Part model, mm, in its own coordinate system. Face numbers are marked on the shaded views. A direction names the side the tool comes from. Round coordinates to 2 decimals unless told otherwise and drop trailing zeros. Loops run counter-clockwise (first coordinate to the right, second up) from the corner with the lowest first, then second, coordinate; pieces in that order, holes last. Notation, with made-up numbers: (40.5, 45) -> (57.5, 45) arc R27 ccw to (57.5, 82) -> close; hole circle Ø6 at (6, 17.5). An arc over 180 degrees is marked (long way). Use a Markdown table: item, result. Add a question column.
Item 1: Flat gauge pins, fed straight in: pin 1 (4 mm diameter, centred on x = 14.5, z = -1.5, fed in from -Y); pin 2 (4 mm diameter, centred on y = 34.5, z = -1, fed in from -X); pin 3 (13.5 mm diameter, centred on x = 0, y = -50, fed in from +Z); pin 4 (1.5 mm diameter, centred on x = -4, z = -1.5, fed in from -Y). Where does each tip first touch, or does it go through?
Item 2: Cut at D-D, the plane y = 54. List the corners of the cut face in (x, z).
Item 3: Cut at A-A, the plane y = 0. List the corners of the cut face in (x, z), plus the area to 3 significant figures.
Item 4: Which spindle directions (+Z, -Z, +X, -X, +Y, -Y) get a long thin tool onto all of the face, cutting with end or side? Do the marked faces 5 and 6. Say none if no direction does.
Item 5: Cut at B-B, the plane x = 41. List the corners of the cut face in (y, z).
Item 6: Two-plate mould, pull along X, no slides. Class the marked faces 1, 2, 3 and 4: pulls with the +X half, pulls with the -X half, needs draft (parallel to the pull), parting line crosses it, or undercut.
Item 7: Cut at C-C, the plane z = 1. State how many separate pieces and enclosed holes the cut face has, plus the area to 3 significant figures.
Item 8: Probe line 1 (Y direction, x = 0, z = 0.75); line 2 (Y direction, x = 0, z = -1.5); line 3 (Y direction, x = 50, z = 1.25). List the from-to ranges inside material, lowest first. Write a range as [from, to].
```python
from build123d import *

# Parameters (mm, degrees)
F0_R        = 11.1
F1_DEPTH    = 3.5
F2_T        = 2.5
F2_T3_DEPTH = 12


# Not quite as in the source:
# - a shell that OpenCascade refuses in one call is made with other operations: the cavity is built on its own and cut out


with BuildPart() as f1:
    # F0 (on Top) → F1 (new body, symmetric)
    with BuildSketch(Plane.XY):
        with BuildLine():
            Line((29.2040910572, 29.1611850262), (15, 50))
            ThreePointArc((15, 50), (0, 35), (-15, 50))
            Line((-15, 50), (-29.2040910572, 29.1611850262))
            Line((-29.2040910572, 29.1611850262), (-50, 15))
            ThreePointArc((-50, 15), (-39.3933982822, 10.6066017178), (-35, 0))
            ThreePointArc((-35, 0), (-39.3933982822, -10.6066017178), (-50, -15))
            Line((-50, -15), (-29.2040910572, -29.1611850262))
            Line((-29.2040910572, -29.1611850262), (-15, -50))
            ThreePointArc((-15, -50), (0, -35), (15, -50))
            Line((15, -50), (29.2040910572, -29.1611850262))
            Line((29.2040910572, -29.1611850262), (50, -15))
            ThreePointArc((50, -15), (35, 0), (50, 15))
            Line((50, 15), (29.2040910572, 29.1611850262))
        make_face()
        Circle(F0_R, mode=Mode.SUBTRACT)
        with BuildLine():
            ThreePointArc((-15, 50), (0, 35), (15, 50))
            ThreePointArc((15, 50), (0, 65), (-15, 50))
        make_face()
        with Locations((0, 50)):
            Circle(F0_R, mode=Mode.SUBTRACT)
        with BuildLine():
            ThreePointArc((65, 0), (60.6066017178, 10.6066017178), (50, 15))
            ThreePointArc((50, 15), (35, 0), (50, -15))
            ThreePointArc((50, -15), (60.6066017178, -10.6066017178), (65, 0))
        make_face()
        with Locations((50, 0)):
            Circle(F0_R, mode=Mode.SUBTRACT)
        with BuildLine():
            ThreePointArc((-15, -50), (0, -65), (15, -50))
            ThreePointArc((15, -50), (0, -35), (-15, -50))
        make_face()
        with Locations((0, -50)):
            Circle(F0_R, mode=Mode.SUBTRACT)
        with BuildLine():
            ThreePointArc((-35, 0), (-39.3933982822, 10.6066017178), (-50, 15))
            ThreePointArc((-50, 15), (-65, 0), (-50, -15))
            ThreePointArc((-50, -15), (-39.3933982822, -10.6066017178), (-35, 0))
        make_face()
        with Locations((-50, 0)):
            Circle(F0_R, mode=Mode.SUBTRACT)
    extrude(amount=F1_DEPTH, both=True)

    # F2: shell of thickness 2.5, made by hand


with BuildPart() as f2_core1:
    # F2_t2: copy of F1
    add(f1.part)

    # the walls: a layer under each face that stays
    f2_faces = [f2_core1.faces().sort_by_distance(p)[0] for p in [
        (39.6020455286, -22.0805925131, 0),
        (22.1020455286, -39.5805925131, 0),
        (0, -65, 0),
        (-22.1020455286, -39.5805925131, 0),
        (-39.6020455286, -22.0805925131, 0),
        (-65, 0, 0),
        (-39.6020455286, 22.0805925131, 0),
        (-22.1020455286, 39.5805925131, 0),
        (0, 65, 0),
        (22.1020455286, 39.5805925131, 0),
        (39.6020455286, 22.0805925131, 0),
        (-61.1, 0, 0),
        (-11.1, -50, 0),
        (38.9, 0, 0),
        (-11.1, 50, 0),
        (-11.1, 0, 0),
        (65, 0, 0),
        (-37.1428571429, -18.5714285714, -3.5),
    ]]
    thicken(f2_faces, amount=-F2_T, mode=Mode.SUBTRACT)

    # F2_s4 → F2_t3 (cut)
    with BuildSketch(Plane.XY.offset(-6)):
        Polygon((50.0140713144, -15.0456639326), (48.5928685595, -12.933606739), (49.2296264469, -12.5), (50, -12.5), align=None)
        Polygon((29.2388199891, -29.1959295426), (27.7969596167, -27.0947917651), (27.4052462259, -27.3615329699), (27.1383293075, -27.753126649), align=None)
        Polygon((15.0456576175, -50.0140805838), (12.9342382503, -48.5919416228), (12.5, -49.2290123454), (12.5, -50), align=None)
        Polygon((-15.0456576175, -50.0140805838), (-12.5, -50), (-12.5, -49.2290123454), (-12.9342382503, -48.5919416228), align=None)
        Polygon((-29.2388199891, -29.1959295426), (-27.1383293075, -27.753126649), (-27.4052462259, -27.3615329699), (-27.7969596167, -27.0947917651), align=None)
        Polygon((-50.0140713144, -15.0456639326), (-48.5928685595, -12.933606739), (-49.2296264469, -12.5), (-50, -12.5), align=None)
        Polygon((-50.0140713144, 15.0456639326), (-50, 12.5), (-49.2296264469, 12.5), (-48.5928685595, 12.933606739), align=None)
        Polygon((-29.2388199891, 29.1959295426), (-27.7969596167, 27.0947917651), (-27.4052462259, 27.3615329699), (-27.1383293075, 27.753126649), align=None)
        Polygon((-15.0456576175, 50.0140805838), (-12.9342382503, 48.5919416228), (-12.5, 49.2290123454), (-12.5, 50), align=None)
        Polygon((15.0456576175, 50.0140805838), (12.5, 50), (12.5, 49.2290123454), (12.9342382503, 48.5919416228), align=None)
        Polygon((29.2388199891, 29.1959295426), (27.1383293075, 27.753126649), (27.4052462259, 27.3615329699), (27.7969596167, 27.0947917651), align=None)
        Polygon((50.0140713144, 15.0456639326), (48.5928685595, 12.933606739), (49.2296264469, 12.5), (50, 12.5), align=None)
    extrude(amount=F2_T3_DEPTH, mode=Mode.SUBTRACT)


with BuildPart() as f1_1:
    add(f1.part)

    # what is left inside the walls is the cavity
    f2_cavity = [f2_core1.part.solids().sort_by_distance(p)[0] for p in [
        (0, -15.95435, 3.475),
    ]]
    add(f2_cavity, mode=Mode.SUBTRACT)


solid = f1_1.part
```
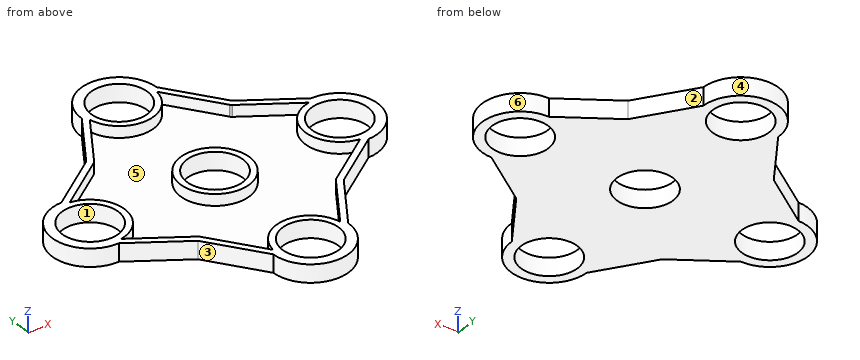
A:
| question | item | result |
|---|---|---|
| 1 | pin 1 | stops at y = -58.29 |
| 1 | pin 2 | stops at x = -26.93 |
| 1 | pin 3 | passes through |
| 1 | pin 4 | stops at y = -64.64 |
| 2 | outline | (-14.46, -3.5) -> (-10.35, -3.5) -> (-10.35, 3.5) -> (-14.46, 3.5) -> close; (10.35, -3.5) -> (14.46, -3.5) -> (14.46, 3.5) -> (10.35, 3.5) -> close |
| 3 | outline | (-65, -3.5) -> (-61.1, -3.5) -> (-61.1, 3.5) -> (-65, 3.5) -> close; (-38.9, -3.5) -> (-11.1, -3.5) -> (-11.1, 3.5) -> (-13.6, 3.5) -> (-13.6, -1) -> (-36.4, -1) -> (-36.4, 3.5) -> (-38.9, 3.5) -> close; (11.1, -3.5) -> (38.9, -3.5) -> (38.9, 3.5) -> (36.4, 3.5) -> (36.4, -1) -> (13.6, -1) -> (13.6, 3.5) -> (11.1, 3.5) -> close; (61.1, -3.5) -> (65, -3.5) -> (65, 3.5) -> (61.1, 3.5) -> close |
| 3 | area | 239 mm^2 |
| 4 | face 5 | +Z |
| 4 | face 6 | +Z, -Z, +X |
| 5 | outline | (-21.13, -3.5) -> (-6.5, -3.5) -> (-6.5, 3.5) -> (-10.2, 3.5) -> (-10.2, -1) -> (-18.1, -1) -> (-18.1, 3.5) -> (-21.13, 3.5) -> close; (6.5, -3.5) -> (21.13, -3.5) -> (21.13, 3.5) -> (18.1, 3.5) -> (18.1, -1) -> (10.2, -1) -> (10.2, 3.5) -> (6.5, 3.5) -> close |
| 6 | face 1 | undercut |
| 6 | face 2 | pulls with the +X half |
| 6 | face 3 | pulls with the -X half |
| 6 | face 4 | parting line crosses it |
| 7 | separate pieces | 2 |
| 7 | enclosed holes | 6 |
| 7 | area | 1,730 mm^2 |
| 8 | line 1 | y = [-65, -61.1], [-38.9, -36.4], [-13.6, -11.1], [11.1, 13.6], [36.4, 38.9], [61.1, 65] |
| 8 | line 2 | y = [-65, -61.1], [-38.9, -11.1], [11.1, 38.9], [61.1, 65] |
| 8 | line 3 | y = [-15, -11.1], [11.1, 15] |
